Input: dimensioned drawing with shaded views. Units: mm. Origin: part minimum x, y, z. A direction names the side the tool comes from. Coordinates: 2 decimals unless noted, no trailing zeros. Order: outer loops, then holes, each group sorted by start corner. A loop starts at its lowest first (then second) coordinate and runs counter-clockwise, first axis right, second up. Notation, with made-up numbers: M 51,86.5 L 106,86.5 A19 ccw 106,109.5 Z; hole C 1.5,11.25 d9. An arc over 180 degrees is marked long. Write item = value, one per line.
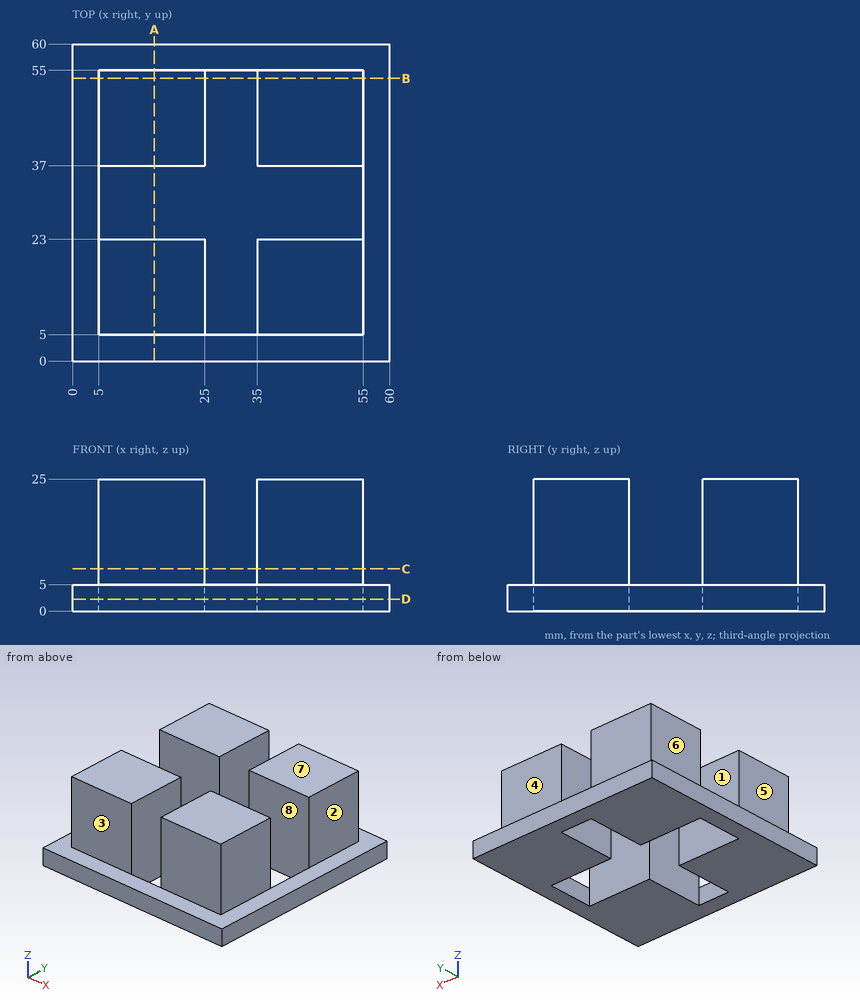
1) Set-up query: the marked faces 1, 2, 3, 4 and 5. Return all of +Z, -Z, +X, -X, +Y, -Y with unobstructed straight access to the full face (end or side cutting, diameter ignored); none if empty.
Numbers:
face_1 = +Z, -Z
face_2 = +Z, +X, +Y, -Y
face_3 = +Z, +X, -X, -Y
face_4 = +Z, +X, -X, +Y
face_5 = +Z, -X, +Y, -Y
2) Section B-B, the plane y = 53.5. Return loops of the section in (x, z).
Numbers:
outline = M 0,0 L 25,0 L 25,25 L 5,25 L 5,5 L 0,5 Z; M 35,0 L 60,0 L 60,5 L 55,5 L 55,25 L 35,25 Z
3) Section D-D, the plane z = 2.25. Return loops of the section in (x, y), and give its area (3 significant figures).
Numbers:
outline = M 0,0 L 60,0 L 60,60 L 0,60 Z; hole M 5,23 L 25,23 L 25,5 L 35,5 L 35,23 L 55,23 L 55,37 L 35,37 L 35,55 L 25,55 L 25,37 L 5,37 Z
area = 2,540 mm²
4) Mould query, pull axis X, two halves, no side actions, for the marked faces 6, 7 and 8. Classes: pulls with the +X half, pulls with the -X half, needs draft (parallel to the pull), parting line crosses it, or undercut.
Numbers:
face_6 = pulls with the -X half
face_7 = needs draft
face_8 = undercut
5) Section A-A, the plane x = 15.5. Return loops of the section in (y, z), and give its area (3 significant figures).
Numbers:
outline = M 0,0 L 23,0 L 23,25 L 5,25 L 5,5 L 0,5 Z; M 37,0 L 60,0 L 60,5 L 55,5 L 55,25 L 37,25 Z
area = 950 mm²
6) Line query: L1, parallel to Y at x = 25.5, z = 2.5; L2, parallel to X at y = 40.5, z = 3.25; L3, parallel to Y at x = 36, z = 3.5. Output: solid intervals per line, ascending.
Numbers:
L1 = 0 to 5, 55 to 60
L2 = 0 to 25, 35 to 60
L3 = 0 to 23, 37 to 60
7) Pin query (flat end, axial travel): pin 1 (2 mm diameter, centred on y = 11, z = 21, fed in from -X); pin 2 (14.5 mm diameter, centred on y = 44.5, z = 15.5, fed in from +X); pin 3 (10 mm diameter, centred on x = 43, z = 10.5, fed in from +Y); pin 4 (6 mm diameter, centred on x = 29.5, z = 7, fed in from +Y). Return the tip coordinate at first contact, or that it passes through.
Numbers:
pin_1 = 5
pin_2 = 55
pin_3 = 55
pin_4 = 60
8) Section C-C, the plane z = 8. Return loops of the section in (x, y), and give its area (3 significant figures).
Numbers:
outline = M 5,5 L 25,5 L 25,23 L 5,23 Z; M 5,37 L 25,37 L 25,55 L 5,55 Z; M 35,5 L 55,5 L 55,23 L 35,23 Z; M 35,37 L 55,37 L 55,55 L 35,55 Z
area = 1,440 mm²
